Can you work these out from the model? Positions are in its coordinate system, mm. A direction names the side the tool comes from. Give positions to 0.01 mm unless a question says otherwise; leave off trailing zeros.
```python
from build123d import *

# Parameters (mm, degrees)
SKETCH1_W              = 300
SKETCH1_H              = 40
BOSS_EXTRUDE1_DEPTH    = 6.35
SKETCH2_W              = 6.35
SKETCH2_H              = 25
BOSS_EXTRUDE2_DEPTH    = 6.35
F_10_CLEARANCE_HOLE1_D = 4.9784
F_8_CLEARANCE_HOLE1_D  = 4.3053
F_6_CLEARANCE_HOLE1_D  = 3.6576


with BuildPart() as part:
    # Sketch1 → Boss-Extrude1 (new body)
    with BuildSketch(Plane(origin=(0, 0, 0), x_dir=(0, 0, -1), z_dir=(1, 0, 0))):
        Rectangle(SKETCH1_W, SKETCH1_H)
    extrude(amount=BOSS_EXTRUDE1_DEPTH)

    # Sketch2 → Boss-Extrude2 (add)
    with BuildSketch(Plane(origin=(6.35, 0, 0), x_dir=(0, 0, -1), z_dir=(1, 0, 0))):
        with Locations((-153.175, 0)):
            Rectangle(SKETCH2_W, SKETCH2_H)
        with Locations((153.175, 0)):
            Rectangle(SKETCH2_W, SKETCH2_H)
    extrude(amount=-BOSS_EXTRUDE2_DEPTH)

    # #10 Clearance Hole1 (through all)
    with Locations(Plane(origin=(6.35, 0, 0), x_dir=(0, 0, -1), z_dir=(1, 0, 0))):
        with Locations((-10, 6.5), (10, 6.5)):
            Hole(F_10_CLEARANCE_HOLE1_D / 2)

    # #8 Clearance Hole1 (through all)
    with Locations(Plane(origin=(6.35, 0, 0), x_dir=(0, 0, -1), z_dir=(1, 0, 0))):
        with Locations((-122, 9), (-98, 9), (-98, -9), (-122, -9), (98, 9), (122, 9), (122, -9), (98, -9)):
            Hole(F_8_CLEARANCE_HOLE1_D / 2)

    # #6 Clearance Hole1 (through all)
    with Locations(Plane(origin=(6.35, 10, 139.5352), x_dir=(0, 0, 1), z_dir=(1, 0, 0))):
        with Locations((0, 0), (0, 20), (-279.0704, 0), (-279.0704, 20)):
            Hole(F_6_CLEARANCE_HOLE1_D / 2)


solid = part.part
```
1) For faces 4 (the face through (3, 12.5, -153)), 5 (the face through (3, 12.5, 153)), 6 (the face through (3, -16, -150)), 7 (the face through (3, -12.5, 153)), which set-ups out of +Z, -Z, +X, -X, +Y, -Y let a thin tool reach every point of the face, with its end or its side?
Values follow:
face 4: -Z, +X, -X, +Y
face 5: +Z, +X, -X, +Y
face 6: -Z, +X, -X, -Y
face 7: +Z, +X, -X, -Y
2) If we mould it in two halves opening along Y, with no side actions, what happens to faces 1 (the face through (3, -12.5, -153)), 2 (the face through (3, 16, -150)), 3 (the face through (3.131, 4.292, 11.149))? For each: +Y half, -Y half, draft (parallel to the pull), parting line (faces both ways), or undercut.
Values follow:
face 1: -Y half
face 2: draft
face 3: undercut
3) For pin 1 Ø1.9 at (x, z) = (4.5, -152.5) entering from -Y; pin 2 Ø3 at (x, y) = (4, 16.5) entering from +Z, each with a flat end and sliding along its axis, tell me the tip position at first contact or that it passes through.
Values follow:
pin 1: stops at y = -12.5
pin 2: stops at z = 150
4) Suppose I cut it at A-A on x = 1.25. State how many separate pieces and enclosed holes the cut face has, plus the area to 3 significant figures.
Values follow:
separate pieces: 1
enclosed holes: 14
area: 12,100 mm2
5) Please list where these lines run through material, in increasing order: L1, parallel to Y at x = 2.75, z = 98; L2, parallel to Z at x = 1, y = 6; L3, parallel to Y at x = 4.75, z = 10.
Values follow:
L1: y = -20 to -11.15, -6.85 to 6.85, 11.15 to 20
L2: z = -156.35 to -12.44, -7.56 to 7.56, 12.44 to 156.35
L3: y = -20 to 4.01, 8.99 to 20
